from build123d import *

# Parameters (mm, degrees)
BOSS_EXTRUDE1_DEPTH = 12
SKETCH2_R           = 1
CUT_EXTRUDE1_DEPTH  = 15
SKETCH4_R           = 2.25
CUT_EXTRUDE3_DEPTH  = 5
SHELL1_DEPTH        = 10
SHELL1_2_DEPTH      = 5
SKETCH3_R           = 9.15
CUT_EXTRUDE2_DEPTH  = 3
FILLET1_R           = 2
BOSS_EXTRUDE2_DEPTH = 7
SKETCH7_W           = 12
SKETCH7_H           = 4.549017994
CUT_EXTRUDE4_DEPTH  = 4
SKETCH8_W           = 27.297760414
SKETCH8_H           = 10.352522689
CUT_EXTRUDE5_DEPTH  = 33
BOSS_EXTRUDE8_DEPTH = 4
SKETCH11_R          = 5.5
CUT_EXTRUDE6_DEPTH  = 4
SKETCH12_R          = 1.5
CUT_EXTRUDE7_DEPTH  = 3
SKETCH13_W          = 0.4
SKETCH13_H          = 1
CUT_EXTRUDE8_DEPTH  = 5
CUT_EXTRUDE9_DEPTH  = 15
FILLET2_R           = 1
BOSS_EXTRUDE9_DEPTH = 4
SKETCH16_R          = 5.25
CUT_EXTRUDE10_DEPTH = 5.1


# Read off the part's stored shape, not the designer's step: Shell1
with BuildPart() as part:
    # Sketch1 → Boss-Extrude1 (new body)
    with BuildSketch(Plane(origin=(0, 0, 0), x_dir=(1, 0, 0), z_dir=(0, 1, 0))):
        with BuildLine():
            Line((-8, 10), (8, 10))
            ThreePointArc((8, 10), (9.414213562, 9.414213562), (10, 8))
            Line((10, 8), (10, -8))
            ThreePointArc((10, -8), (9.414213562, -9.414213562), (8, -10))
            Line((8, -10), (-8, -10))
            ThreePointArc((-8, -10), (-9.414213562, -9.414213562), (-10, -8))
            Line((-10, -8), (-10, 8))
            ThreePointArc((-10, 8), (-9.414213562, 9.414213562), (-8, 10))
        make_face()
    extrude(amount=BOSS_EXTRUDE1_DEPTH)

    # Sketch2 → Cut-Extrude1 (cut)
    with BuildSketch(Plane.XZ):
        with Locations(Location((-8.5, 8.5, 0), (0, 0, 270))):
            Circle(SKETCH2_R)
        with Locations(Location((8.5, 8.5, 0), (0, 0, 270))):
            Circle(SKETCH2_R)
        with Locations(Location((8.5, -8.5, 0), (0, 0, 270))):
            Circle(SKETCH2_R)
        with Locations(Location((-8.5, -8.5, 0), (0, 0, 270))):
            Circle(SKETCH2_R)
    extrude(amount=-CUT_EXTRUDE1_DEPTH, mode=Mode.SUBTRACT)

    # Sketch4 → Cut-Extrude3 (cut)
    with BuildSketch(Plane(origin=(0, 12, 0), x_dir=(1, 0, 0), z_dir=(0, 1, 0))):
        with Locations((8.5, -8.5)):
            Circle(SKETCH4_R)
        with Locations((-8.5, -8.5)):
            Circle(SKETCH4_R)
        with Locations((-8.5, 8.5)):
            Circle(SKETCH4_R)
        with Locations((8.5, 8.5)):
            Circle(SKETCH4_R)
    extrude(amount=-CUT_EXTRUDE3_DEPTH, mode=Mode.SUBTRACT)

    # Shell1 outline → Shell1 (cut)
    with BuildSketch(Plane(origin=(0, 0, 0), x_dir=(1, 0, 0), z_dir=(0, 1, 0))):
        with BuildLine():
            Line((-4.279514246, -8), (4.279514246, -8))
            ThreePointArc((4.279514246, -8), (5.49479618, -5.49479618), (8, -4.279514246))
            Line((8, -4.279514246), (8, 4.279514246))
            ThreePointArc((8, 4.279514246), (5.49479618, 5.49479618), (4.279514246, 8))
            Line((4.279514246, 8), (-4.279514246, 8))
            ThreePointArc((-4.279514246, 8), (-5.49479618, 5.49479618), (-8, 4.279514246))
            Line((-8, 4.279514246), (-8, -4.279514246))
            ThreePointArc((-8, -4.279514246), (-5.49479618, -5.49479618), (-4.279514246, -8))
        make_face()
    extrude(amount=SHELL1_DEPTH, mode=Mode.SUBTRACT)

    # Shell1 2 outline → Shell1 2 (cut)
    with BuildSketch(Plane(origin=(0, 0, 0), x_dir=(1, 0, 0), z_dir=(0, 1, 0))):
        with BuildLine():
            Line((4.279514246, -8), (5.541960108, -8))
            ThreePointArc((5.541960108, -8), (6.378679656, -6.378679656), (8, -5.541960108))
            Line((8, -5.541960108), (8, -4.279514246))
            ThreePointArc((8, -4.279514246), (5.49479618, -5.49479618), (4.279514246, -8))
        make_face()
        with BuildLine():
            Line((-5.541960108, -8), (-4.279514246, -8))
            ThreePointArc((-4.279514246, -8), (-5.49479618, -5.49479618), (-8, -4.279514246))
            Line((-8, -4.279514246), (-8, -5.541960108))
            ThreePointArc((-8, -5.541960108), (-6.378679656, -6.378679656), (-5.541960108, -8))
        make_face()
        with BuildLine():
            ThreePointArc((4.279514246, 8), (5.49479618, 5.49479618), (8, 4.279514246))
            Line((8, 4.279514246), (8, 5.541960108))
            ThreePointArc((8, 5.541960108), (6.378679656, 6.378679656), (5.541960108, 8))
            Line((5.541960108, 8), (4.279514246, 8))
        make_face()
        with BuildLine():
            Line((-8, 5.541960108), (-8, 4.279514246))
            ThreePointArc((-8, 4.279514246), (-5.49479618, 5.49479618), (-4.279514246, 8))
            Line((-4.279514246, 8), (-5.541960108, 8))
            ThreePointArc((-5.541960108, 8), (-6.378679656, 6.378679656), (-8, 5.541960108))
        make_face()
    extrude(amount=SHELL1_2_DEPTH, mode=Mode.SUBTRACT)

    # Sketch3 → Cut-Extrude2 (cut)
    with BuildSketch(Plane.XZ):
        Circle(SKETCH3_R)
    extrude(amount=-CUT_EXTRUDE2_DEPTH, mode=Mode.SUBTRACT)

    # Fillet1
    fillet1_edges = [part.edges().sort_by_distance(p)[0] for p in [
        (6.822949017, 9.5, -10),
        (10, 9.5, -6.822949017),
        (-6.822949017, 9.5, -10),
        (-10, 9.5, -6.822949017),
        (-10, 9.5, 6.822949017),
        (-6.822949017, 9.5, 10),
        (6.822949017, 9.5, 10),
        (10, 9.5, 6.822949017),
    ]]
    fillet(fillet1_edges, radius=FILLET1_R)

    # Sketch6 → Boss-Extrude2 (add)
    with BuildSketch(Plane.XZ):
        with BuildLine():
            Line((-7.5, -10), (7.5, -10))
            Line((7.5, -10), (7.5, -14))
            ThreePointArc((7.5, -14), (6.914213562, -15.414213562), (5.5, -16))
            Line((5.5, -16), (-5.5, -16))
            ThreePointArc((-5.5, -16), (-6.914213562, -15.414213562), (-7.5, -14))
            Line((-7.5, -14), (-7.5, -10))
        make_face()
    extrude(amount=-BOSS_EXTRUDE2_DEPTH)

    # Sketch7 → Cut-Extrude4 (cut)
    with BuildSketch(Plane.XZ):
        with Locations((0, -13.725491003)):
            Rectangle(SKETCH7_W, SKETCH7_H)
    extrude(amount=-CUT_EXTRUDE4_DEPTH, mode=Mode.SUBTRACT)

    # Sketch8 → Cut-Extrude5 (cut)
    with BuildSketch(Plane(origin=(10, 0, 0), x_dir=(0, 0, -1), z_dir=(1, 0, 0))):
        with Locations((3.648880207, 12.176261345)):
            Rectangle(SKETCH8_W, SKETCH8_H)
    extrude(amount=-CUT_EXTRUDE5_DEPTH, mode=Mode.SUBTRACT)

    # Sketch10 → Boss-Extrude8 (add)
    with BuildSketch(Plane(origin=(0, 7, 0), x_dir=(1, 0, 0), z_dir=(0, 1, 0))):
        Polygon((9.294915126, 4.441002139), (-9.072540785, 4.441002139), (-5.843708737, 9.485613806), (6.066083078, 9.485613806), align=None)
    extrude(amount=-BOSS_EXTRUDE8_DEPTH)

    # Sketch11 → Cut-Extrude6 (cut)
    with BuildSketch(Plane.XZ.offset(-3)):
        Circle(SKETCH11_R)
    extrude(amount=-CUT_EXTRUDE6_DEPTH, mode=Mode.SUBTRACT)

    # Sketch12 → Cut-Extrude7 (cut)
    with BuildSketch(Plane(origin=(0, 7, 0), x_dir=(1, 0, 0), z_dir=(0, 1, 0))):
        with Locations(Location((0, 7.75, 0), (0, 0, 270))):
            Circle(SKETCH12_R)
    extrude(amount=-CUT_EXTRUDE7_DEPTH, mode=Mode.SUBTRACT)

    # Sketch13 → Cut-Extrude8 (cut)
    with BuildSketch(Plane(origin=(0, 4, 0), x_dir=(1, 0, 0), z_dir=(0, 1, 0))):
        with Locations((0, 7.75)):
            Rectangle(SKETCH13_W, SKETCH13_H)
    extrude(amount=-CUT_EXTRUDE8_DEPTH, mode=Mode.SUBTRACT)

    # Sketch14 → Cut-Extrude9 (cut)
    with BuildSketch(Plane(origin=(0, 7, 0), x_dir=(1, 0, 0), z_dir=(0, 1, 0))):
        with BuildLine():
            Line((-5, 14.5), (5, 14.5))
            ThreePointArc((5, 14.5), (5.707106781, 14.207106781), (6, 13.5))
            Line((6, 13.5), (6, 11))
            ThreePointArc((6, 11), (5.707106781, 10.292893219), (5, 10))
            Line((5, 10), (-5, 10))
            ThreePointArc((-5, 10), (-5.707106781, 10.292893219), (-6, 11))
            Line((-6, 11), (-6, 13.5))
            ThreePointArc((-6, 13.5), (-5.707106781, 14.207106781), (-5, 14.5))
        make_face()
    extrude(amount=-CUT_EXTRUDE9_DEPTH, mode=Mode.SUBTRACT)

    # Fillet2
    fillet2_edges = [part.edges().sort_by_distance(p)[0] for p in [
        (-6, 4, -14.718245837),
        (6, 4, -14.718245837),
    ]]
    fillet(fillet2_edges, radius=FILLET2_R)

    # Sketch15 → Boss-Extrude9 (add)
    with BuildSketch(Plane(origin=(0, 7, 0), x_dir=(1, 0, 0), z_dir=(0, 1, 0))):
        Polygon((4.927887467, -8.83937155), (8.987059624, -4.361499915), (8.535312268, 4.849371277), (4.119785389, 6.639048991), (-3.498767695, 5.109974325), (-8.089855619, 5.874511658), (-8.702967098, -5.068680896), (-4.41401834, -8.956595244), align=None)
    extrude(amount=-BOSS_EXTRUDE9_DEPTH)

    # Sketch16 → Cut-Extrude10 (cut)
    with BuildSketch(Plane(origin=(0, 7, 0), x_dir=(1, 0, 0), z_dir=(0, 1, 0))):
        with Locations(Location((0, 0, 0), (0, 0, 270))):
            Circle(SKETCH16_R)
    extrude(amount=-CUT_EXTRUDE10_DEPTH, mode=Mode.SUBTRACT)


solid = part.part
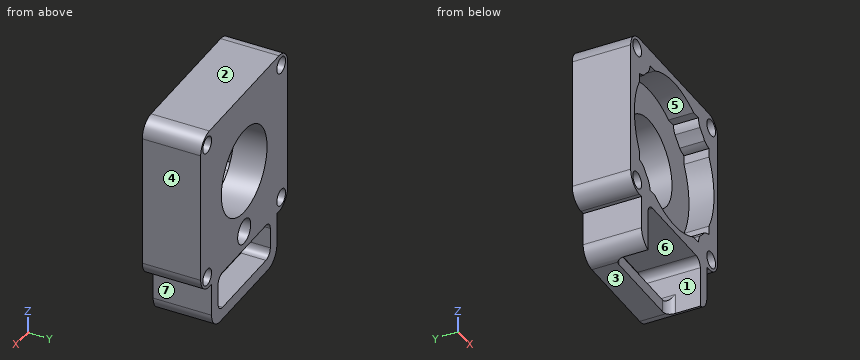
Part model, mm, in its own coordinate system. Face numbers are marked on the shaded views. A direction names the side the tool comes from. Coordinates: 2 decimals unless noted, no trailing zeros. Write each loop counter-clockwise with the first axis right and the second up, starting at its lowest first coordinate (ties: lowest second). Pieces come first, ordered by that corner, then holes. Notation, with made-up numbers: M 82,51.5 L 94,51.5 A16 ccw 94,81.5 Z; hole C 40,-25.75 d1. An arc over 180 degrees is marked long. Return JSON: item names as keys, results as strings.
1. Saw through at D-D, the plane z = 8.5. Write the cut outline in (x, y), then the cut area to 3 significant figures.
Determined:
{"outline": "M -9.94,0 L -9.5,0 L -9.5,7 L -9.94,7 Z; M -7.5,0 L -3.39,0 L -3.39,3 L 3.39,3 L 3.39,0 L 7.5,0 L 7.5,7 L -7.5,7 Z; M 9.5,0 L 9.94,0 L 9.94,7 L 9.5,7 Z", "area": "90.8 mm²"}
2. Flat gauge pins, fed straight in: pin 1 Ø1.6 at (x, z) = (-1.5, -15) entering from -Y; pin 2 Ø0.9 at (x, y) = (5, 2) entering from -Z; pin 3 Ø1.8 at (x, z) = (8.5, 8.5) entering from -Y; pin 4 Ø3 at (y, z) = (3.5, -11) entering from +X. Where does each tip first touch, or does it go through?
Determined:
{"pin 1": "y = 4", "pin 2": "z = -10.11", "pin 3": "through", "pin 4": "x = 9.32"}
3. Saw through at C-C, the plane y = 6.5. Write the cut outline in (x, z), then the cut area to 3 significant figures.
Determined:
{"outline": "M -10,-8 A2 ccw -8,-10 L -7.5,-10 L -7.5,-14 A2 ccw -5.5,-16 L 5.5,-16 A2 ccw 7.5,-14 L 7.5,-10 L 8,-10 A2 ccw 10,-8 L 10,8 A2 ccw 8,10 L -8,10 A2 ccw -10,8 Z; hole C -8.5,-8.5 d2; hole C -8.5,8.5 d2; hole M -6,-13.5 A1 ccw -5,-14.5 L 5,-14.5 A1 ccw 6,-13.5 L 6,-11 A1 ccw 5,-10 L -5,-10 A1 ccw -6,-11 Z; hole C 0,0 d10.5; hole C 0,-7.75 d3; hole C 8.5,-8.5 d2; hole C 8.5,8.5 d2", "area": "325 mm²"}
4. Saw through at B-B, the plane x = -2.75. Write the cut outline in (y, z), then the cut area to 3 significant figures.
Determined:
{"outline": "M 0,-10 L 7,-10 L 7,-4.47 L 3,-4.47 L 3,-8.73 L 0,-8.73 Z; M 0,8.73 L 3,8.73 L 3,4.47 L 7,4.47 L 7,10 L 0,10 Z; M 4,-16 L 7,-16 L 7,-14.5 L 4,-14.5 Z", "area": "56.4 mm²"}
5. Pull direction Z, two halves, no side cores. Call the marked faces 1, 2, 3 and 4: pulls with the +Z half, pulls with the -Z half, needs draft (parallel to the pull), parting line crosses it, or undercut.
Determined:
{"face 1": "undercut", "face 2": "pulls with the +Z half", "face 3": "pulls with the -Z half", "face 4": "needs draft"}
6. 3-axis set-ups, long thin cutter, end or side, ignore diameter. For the marked faces 5, 6 and 7: which of +Z, -Z, +X, -X, +Y, -Y reach the whole face in a straight line?
Determined:
{"face 5": "-Y", "face 6": "+Y, -Y", "face 7": "-Z, +X, +Y, -Y"}
7. Saw through at A-A, the plane z = 0. Write the cut outline in (x, y).
Determined:
{"outline": "M -10,0 L -9.15,0 L -9.15,3 L -5.25,3 L -5.25,7 L -10,7 Z; M 5.25,3 L 9.15,3 L 9.15,0 L 10,0 L 10,7 L 5.25,7 Z"}
8. Probe L1, parallel to X at y = 2.75, z = -14; L2, parallel to X at y = 4.5, z = -8.5; L3, parallel to X at y = 5.65, z = -7.75. List the from-to ranges inside material, lowest first.
Determined:
{"L1": "-7.5 to -6, 6 to 7.5", "L2": "-9.94 to -9.5, -7.5 to -1.3, 1.3 to 7.5, 9.5 to 9.94", "L3": "-10 to -9.16, -7.84 to -1.5, 1.5 to 7.84, 9.16 to 10"}
